```python
from build123d import *

# Parameters (mm, degrees)
F0_W     = 84.7769677639
F0_H     = 43.2662777603
F1_DEPTH = 4.3966565281
F2_W     = 84.4204500318
F2_H     = 9.8768174648
F3_DEPTH = 31.4335487783
F4_W     = 86.0934257507
F4_H     = 8.3434134722
F5_DEPTH = 31.7156463861
F6_W     = 10.8002573252
F6_H     = 39.9001836777
F7_DEPTH = 30.848281458


with BuildPart() as f1:
    # F0 (on Top) → F1 (new body)
    with BuildSketch(Plane.XY):
        with Locations((-42.388483882, -21.6331388801)):
            Rectangle(F0_W, F0_H)
    extrude(amount=F1_DEPTH)

    # F2 (on Top) → F3 (join)
    with BuildSketch(Plane.XY):
        with Locations((-42.2102250159, 4.9384087324)):
            Rectangle(F2_W, F2_H)
    extrude(amount=F3_DEPTH)

    # F4 (on Top) → F5 (join)
    with BuildSketch(Plane.XY):
        with Locations((-43.0467128754, -46.2585315108)):
            Rectangle(F4_W, F4_H)
    extrude(amount=F5_DEPTH)

    # F6 (on Top) → F7 (join)
    with BuildSketch(Plane.XY):
        with Locations((-5.4001286626, -19.9500918388)):
            Rectangle(F6_W, F6_H)
    extrude(amount=F7_DEPTH)


solid = f1.part
```
Build history of the part. All positions in model axes, mm. A direction names the side the tool comes from. Round coordinates to 2 decimals unless told otherwise and drop trailing zeros. Loops run counter-clockwise (first coordinate to the right, second up) from the corner with the lowest first, then second, coordinate; pieces in that order, holes last.
Item 1: Saw through at B-B (x = -7). List the corners of the cut face in (y, z).
Item 2: Saw through at A-A (z = 10). List the corners of the cut face in (x, y), then the cut area to 3 significant figures.
Item 3: Drill centre lines: line 1 along Y through (x, z) = (-49.5, 26); line 2 along X through (y, z) = (-36, 6); line 3 along X through (y, z) = (-34, 3). Where is each one in solid material? Low to high.
Item 4: Two-plate mould, pull along Y, no slides. Class faces 5 (the face through (-10.8, -20, 17)), 6 (the face through (-52, 0, 18)), 7 (the face through (-44, -46, 31.716)), 8 (the face through (-44, -50.43, 16)): released by +Y, released by -Y, zero draft, split by the parting line, or undercut.
Item 5: Pin check, flat tips, straight feed: P1, Ø4, axis at x = -42.5, y = -29.5, coming from the +Z side; P2, Ø6, axis at y = -20, z = 8, coming from the -X side; P3, Ø12, axis at x = -4, y = -24.5, coming from the +Z side; P4, Ø1.5, axis at x = -68, y = -26.5, coming from the -Z side. Stop position of each tip, or through.
Item 6: Saw through at C-C (y = -4). List the corners of the cut face in (x, z), then the cut area to 3 significant figures.
Item 7: Which spindle directions (+Z, -Z, +X, -X, +Y, -Y) get a long thin tool onto all of the face, cutting with end or side? Do faces 1 (the face through (-44, -20, 0)), 2 (the face through (-5, -39.9, 17)), 3 (the face through (-84.777, -21, 2)), 4 (the face through (-43, 5, 31.434)). Say none if no direction does.
Item 8: Saw through at D-D (x = -50.5). List the corners of the cut face in (y, z), then the cut area to 3 significant figures.
Worked answers:
1. outline: (-50.43, 0) - (9.88, 0) - (9.88, 31.43) - (0, 31.43) - (0, 30.85) - (-39.9, 30.85) - (-39.9, 4.4) - (-42.09, 4.4) - (-42.09, 31.72) - (-50.43, 31.72) - close
2. outline: (-86.09, -50.43) - (0, -50.43) - (0, -42.09) - (-86.09, -42.09) - close; (-84.42, 0) - (-10.8, 0) - (-10.8, -39.9) - (0, -39.9) - (0, 9.88) - (-84.42, 9.88) - close
2. area: 1,980 mm2
3. line 1: y = -50.43 to -42.09, 0 to 9.88
3. line 2: x = -10.8 to 0
3. line 3: x = -84.78 to 0
4. face 5: undercut
4. face 6: undercut
4. face 7: zero draft
4. face 8: released by -Y
5. P1: stops at z = 4.4
5. P2: stops at x = -10.8
5. P3: stops at z = 30.85
5. P4: stops at z = 0
6. outline: (-84.78, 0) - (0, 0) - (0, 30.85) - (-10.8, 30.85) - (-10.8, 4.4) - (-84.78, 4.4) - close
6. area: 658 mm2
7. face 1: -Z, +X, -X, +Y, -Y
7. face 2: +Z, +X, -X
7. face 3: +Z, -Z, -X, +Y
7. face 4: +Z, +X, -X, +Y
8. outline: (-50.43, 0) - (9.88, 0) - (9.88, 31.43) - (0, 31.43) - (0, 4.4) - (-42.09, 4.4) - (-42.09, 31.72) - (-50.43, 31.72) - close
8. area: 760 mm2
